Design review of the part built by this model. Coordinates are the model's own, in mm. A direction names the side the tool comes from. Coordinates: 2 decimals unless noted, no trailing zeros. Write each loop counter-clockwise with the first axis right and the second up, starting at its lowest first coordinate (ties: lowest second). Pieces come first, ordered by that corner, then holes.
Q1. Add section B-B, the plane z = 1.4. Give the boundary of the cut face in (x, y).
Q2. Machinability: for faces 4 (the face through (10.535, 4.35, 1.479)), 5 (the face through (0, -4, 3)), which of the approach directions +Z, -Z, +X, -X, +Y, -Y give a long, thin tool a straight path to every point of the face, cutting with its end or side? Answer none if there is none.
Q3. Clearance check with flat-ended pins moving along their axes: pin 1 Ø5 at (x, y) = (-13, 0) entering from -Z; pin 2 Ø1 at (y, z) = (16.5, 1.5) entering from -X; pin 3 Ø1.5 at (y, z) = (9.5, 1.5) entering from +X; pin 4 Ø1 at (y, z) = (-5, 2.5) entering from +X. State where each tip first meets the part, or that it passes through.
Q4. Add section A-A, the plane x = 0. Give the boundary of the cut face in (y, z), plus the area to 3 significant figures.
Q5. The part is to be moulded in two halves that separate along X. For faces 1 (the face through (10.465, -4.31, 1.479)), 2 (the face through (-4.444, -20.013, 1.479)), 3 (the face through (0, -4, 0)), say which applies: +X half, -X half, draft (parallel to the pull), parting line (faces both ways), or undercut.
Q6. To check wall thickness, follow probe 1 along Y at (x, z) = (0, 0.8); probe 2 along X at (y, z) = (5, 1.2); probe 3 along Y at (x, z) = (-14, 1.55). State the ranges of each line that lie inside material, in increasing order.
Q7. Add section D-D, the plane x = -12.5. Give the boundary of the cut face in (y, z).
Q8. Add section C-C, the plane y = 0. Give the boundary of the cut face in (x, z).
from build123d import *

# Parameters (mm, degrees)
SKETCH1_R           = 20.5
SKETCH1_R_2         = 3
SKETCH1_R_3         = 1.5
BOSS_EXTRUDE1_DEPTH = 3


with BuildPart() as part:
    # Sketch1 → Boss-Extrude1 (new body)
    with BuildSketch(Plane.XY):
        Circle(SKETCH1_R)
        with Locations((-13, 0)):
            Circle(SKETCH1_R_2, mode=Mode.SUBTRACT)
        Circle(SKETCH1_R_3, mode=Mode.SUBTRACT)
        Polygon((18, 2.886751346), (13, 5.773502692), (8, 2.886751346), (8, -2.886751346), (13, -5.773502692), (18, -2.886751346), align=None, mode=Mode.SUBTRACT)
    extrude(amount=BOSS_EXTRUDE1_DEPTH)


solid = part.part
Here are the results:
1. outline: circle Ø41 at (0, 0); hole circle Ø6 at (-13, 0); hole circle Ø3 at (0, 0); hole (8, -2.89) - (13, -5.77) - (18, -2.89) - (18, 2.89) - (13, 5.77) - (8, 2.89) - close
2. face 4: +Z, -Z
2. face 5: +Z, +X, -X, +Y, -Y
3. pin 1: passes through
3. pin 2: stops at x = -12.82
3. pin 3: stops at x = 18.54
3. pin 4: stops at x = 20
4. outline: (-20.5, 0) - (-1.5, 0) - (-1.5, 3) - (-20.5, 3) - close; (1.5, 0) - (20.5, 0) - (20.5, 3) - (1.5, 3) - close
4. area: 114 mm2
5. face 1: undercut
5. face 2: parting line
5. face 3: draft
6. probe 1: y = -20.5 to -1.5, 1.5 to 20.5
6. probe 2: x = -19.88 to 11.66, 14.34 to 19.88
6. probe 3: y = -14.97 to -2.83, 2.83 to 14.97
7. outline: (-16.25, 0) - (-2.96, 0) - (-2.96, 3) - (-16.25, 3) - close; (2.96, 0) - (16.25, 0) - (16.25, 3) - (2.96, 3) - close
8. outline: (-20.5, 0) - (-16, 0) - (-16, 3) - (-20.5, 3) - close; (-10, 0) - (-1.5, 0) - (-1.5, 3) - (-10, 3) - close; (1.5, 0) - (8, 0) - (8, 3) - (1.5, 3) - close; (18, 0) - (20.5, 0) - (20.5, 3) - (18, 3) - close
